```python
from build123d import *

# Parameters (mm, degrees)
F0_R     = 6
F1_DEPTH = 2.5
F2_W     = 98
F2_H     = 52
F3_DEPTH = 25


with BuildPart() as f1:
    # F0 (on Top) → F1 (new body)
    with BuildSketch(Plane.XY):
        with BuildLine():
            Line((98.5, 54.5), (-0.5, 54.5))
            ThreePointArc((-0.5, 54.5), (-1.9142135624, 53.9142135624), (-2.5, 52.5))
            Line((-2.5, 52.5), (-2.5, -0.5))
            ThreePointArc((-2.5, -0.5), (-1.9142135624, -1.9142135624), (-0.5, -2.5))
            Line((-0.5, -2.5), (98.5, -2.5))
            ThreePointArc((98.5, -2.5), (99.9142135624, -1.9142135624), (100.5, -0.5))
            Line((100.5, -0.5), (100.5, 52.5))
            ThreePointArc((100.5, 52.5), (99.9142135624, 53.9142135624), (98.5, 54.5))
        make_face()
        Polygon((22, 0), (0, 0), (0, 52), (98, 52), (98, 0), align=None, mode=Mode.SUBTRACT)
        Polygon((0, 52), (0, 0), (22, 0), (98, 0), (98, 52), align=None)
        with BuildLine():
            ThreePointArc((24.5, 2.5), (23.767766953, 0.732233047), (22, 0))
            ThreePointArc((22, 0), (20.232233047, 4.267766953), (24.5, 2.5))
        make_face(mode=Mode.SUBTRACT)
        with Locations((88, 44)):
            Circle(F0_R, mode=Mode.SUBTRACT)
    extrude(amount=F1_DEPTH)

    # F2 (on Top) → F3 (join)
    with BuildSketch(Plane.XY):
        with BuildLine():
            Line((98.5, 54.5), (-0.5, 54.5))
            ThreePointArc((-0.5, 54.5), (-1.9142135624, 53.9142135624), (-2.5, 52.5))
            Line((-2.5, 52.5), (-2.5, -0.5))
            ThreePointArc((-2.5, -0.5), (-1.9142135624, -1.9142135624), (-0.5, -2.5))
            Line((-0.5, -2.5), (98.5, -2.5))
            ThreePointArc((98.5, -2.5), (99.9142135624, -1.9142135624), (100.5, -0.5))
            Line((100.5, -0.5), (100.5, 52.5))
            ThreePointArc((100.5, 52.5), (99.9142135624, 53.9142135624), (98.5, 54.5))
        make_face()
        with Locations((49, 26)):
            Rectangle(F2_W, F2_H, mode=Mode.SUBTRACT)
    extrude(amount=-F3_DEPTH)


solid = f1.part
```
The model under review builds one solid part; all positions refer to its coordinate system, in mm. A direction names the side the tool comes from. Round coordinates to 2 decimals unless told otherwise and drop trailing zeros. Loops run counter-clockwise (first coordinate to the right, second up) from the corner with the lowest first, then second, coordinate; pieces in that order, holes last.
1) Consider section B-B on z = -1. State the section outline as (x, y) points.
Values follow:
outline: (-2.5, -0.5) arc R2 ccw to (-0.5, -2.5) - (98.5, -2.5) arc R2 ccw to (100.5, -0.5) - (100.5, 52.5) arc R2 ccw to (98.5, 54.5) - (-0.5, 54.5) arc R2 ccw to (-2.5, 52.5) - close; hole (0, 0) - (98, 0) - (98, 52) - (0, 52) - close
2) Consider section D-D on x = 67. State the section outline as (y, z) points.
Values follow:
outline: (-2.5, -25) - (0, -25) - (0, 0) - (52, 0) - (52, -25) - (54.5, -25) - (54.5, 2.5) - (-2.5, 2.5) - close
3) Consider section A-A on x = 88. State the section outline as (y, z) points, then the cut area to 4 significant figures.
Values follow:
outline: (-2.5, -25) - (0, -25) - (0, 0) - (38, 0) - (38, 2.5) - (-2.5, 2.5) - close; (50, 0) - (52, 0) - (52, -25) - (54.5, -25) - (54.5, 2.5) - (50, 2.5) - close
area: 237.5 mm2
4) The part is to be moulded in two halves that separate along X. For faces 3 (the face through (99.9, -1.93, -11.06)), 4 (the face through (0, 26, -12)), 5 (the face through (-1.9, 53.93, -11.06)), say which applies: pulls with the +X half, pulls with the -X half, needs draft (parallel to the pull), parting line crosses it, or undercut.
Values follow:
face 3: pulls with the +X half
face 4: undercut
face 5: pulls with the -X half
5) Clearance check with flat-ended pins moving along their axes: P1, Ø8, axis at x = 90, y = 40, coming from the -Z side; P2, Ø6, axis at x = 22, y = 2.5, coming from the +Z side; P3, Ø11, axis at x = 88, y = 44, coming from the -Z side. State where each tip first meets the part, or that it passes through.
Values follow:
P1: stops at z = 0
P2: stops at z = 2.5
P3: passes through
6) Wall thickness on line 1 along X through (y, z) = (34, -15); line 2 along Y through (x, z) = (6, -20.25); line 3 along Y through (x, z) = (22, 1.8): over which ranges is each line inside the solid? List them lowest first.
Values follow:
line 1: x = -2.5 to 0, 98 to 100.5
line 2: y = -2.5 to 0, 52 to 54.5
line 3: y = -2.5 to 0, 5 to 54.5
7) Consider section C-C on y = 44. State the section outline as (x, z) points.
Values follow:
outline: (-2.5, -25) - (0, -25) - (0, 0) - (82, 0) - (82, 2.5) - (-2.5, 2.5) - close; (94, 0) - (98, 0) - (98, -25) - (100.5, -25) - (100.5, 2.5) - (94, 2.5) - close
8) Tool access review of faces 1 (the face through (48, -2.5, -11)), 2 (the face through (48, 26, 0)): name each direction out of +Z, -Z, +X, -X, +Y, -Y from which nothing blocks a thin tool from reaching the whole face with its end or side.
Values follow:
face 1: +Z, -Z, +X, -X, -Y
face 2: -Z
